from build123d import *

# Parameters (mm, degrees)
SKETCH2_W           = 250
SKETCH2_H           = 250
BOSS_EXTRUDE1_DEPTH = 3.175
SKETCH10_W          = 45
SKETCH10_H          = 3.175
BOSS_EXTRUDE2_DEPTH = 12.5
SKETCH11_W          = 45
SKETCH11_H          = 3.175
BOSS_EXTRUDE3_DEPTH = 12.5
SKETCH13_W          = 45
SKETCH13_H          = 3.175
BOSS_EXTRUDE4_DEPTH = 12.5
SKETCH14_W          = 45
SKETCH14_H          = 3.175
BOSS_EXTRUDE5_DEPTH = 12.5
M3_TAPPED_HOLE1_D   = 2.5
SKETCH21_R          = 1.25
CUT_EXTRUDE2_DEPTH  = 10
SKETCH23_R          = 2.9718
CUT_EXTRUDE10_DEPTH = 10


with BuildPart() as part:
    # Sketch2 → Boss-Extrude1 (new body)
    with BuildSketch(Plane(origin=(0, 0, 0), x_dir=(1, 0, 0), z_dir=(0, 1, 0))):
        Rectangle(SKETCH2_W, SKETCH2_H)
    extrude(amount=BOSS_EXTRUDE1_DEPTH)

    # Sketch10 → Boss-Extrude2 (add)
    with BuildSketch(Plane(origin=(0, 0, -125), x_dir=(-1, 0, 0), z_dir=(0, 0, -1))):
        with Locations((0, 1.5875)):
            Rectangle(SKETCH10_W, SKETCH10_H)
    extrude(amount=BOSS_EXTRUDE2_DEPTH)

    # Sketch11 → Boss-Extrude3 (add)
    with BuildSketch(Plane.ZY.offset(125)):
        with Locations((0, 1.5875)):
            Rectangle(SKETCH11_W, SKETCH11_H)
    extrude(amount=BOSS_EXTRUDE3_DEPTH)

    # Sketch13 → Boss-Extrude4 (add)
    with BuildSketch(Plane.XY.offset(125)):
        with Locations((0, 1.5875)):
            Rectangle(SKETCH13_W, SKETCH13_H)
    extrude(amount=BOSS_EXTRUDE4_DEPTH)

    # Sketch14 → Boss-Extrude5 (add)
    with BuildSketch(Plane(origin=(125, 0, 0), x_dir=(0, 0, -1), z_dir=(1, 0, 0))):
        with Locations((0, 1.5875)):
            Rectangle(SKETCH14_W, SKETCH14_H)
    extrude(amount=BOSS_EXTRUDE5_DEPTH)

    # M3 Tapped Hole1 (through all)
    with Locations(Plane(origin=(-115, 3.175, -115), x_dir=(0, 0, 1), z_dir=(0, 1, 0))):
        with Locations((0, 0)):
            Hole(M3_TAPPED_HOLE1_D / 2)

    # Sketch21 → Cut-Extrude2 (cut)
    with BuildSketch(Plane(origin=(0, 3.175, 0), x_dir=(1, 0, 0), z_dir=(0, 1, 0))):
        with Locations((115, 115)):
            Circle(SKETCH21_R)
        with Locations((115, -115)):
            Circle(SKETCH21_R)
        with Locations((-115, -115)):
            Circle(SKETCH21_R)
    extrude(amount=-CUT_EXTRUDE2_DEPTH, mode=Mode.SUBTRACT)

    # Sketch23 → Cut-Extrude10 (cut)
    with BuildSketch(Plane(origin=(0, 3.175, 0), x_dir=(1, 0, 0), z_dir=(0, 1, 0))):
        with Locations((-70.403440877, -69.85)):
            Circle(SKETCH23_R)
        with Locations((-70.403440877, 69.85)):
            Circle(SKETCH23_R)
        with Locations((69.296559123, 69.85)):
            Circle(SKETCH23_R)
        with Locations((69.296559123, -69.85)):
            Circle(SKETCH23_R)
    extrude(amount=-CUT_EXTRUDE10_DEPTH, mode=Mode.SUBTRACT)


solid = part.part
The model under review builds one solid part; all positions refer to its coordinate system, in mm. Round coordinates to 2 decimals unless told otherwise and drop trailing zeros. Loops run counter-clockwise (first coordinate to the right, second up) from the corner with the lowest first, then second, coordinate; pieces in that order, holes last. Notation, with made-up numbers: (36.25, -34.75) -> (41.25, -34.75) arc R20 ccw to (41.25, -12.75) -> close; hole circle Ø1 at (-15.75, -22). An arc over 180 degrees is marked (long way). Return JSON: item names as keys, results as strings.
(1) The part is to be moulded in two halves that separate along Z. For faces 1 (the cylindrical face through (-67.66, 1.61, 70.99)), 2 (the flat face through (-2, 3.175, -2)), say which applies: released by +Z, released by -Z, zero draft, split by the parting line, or undercut.
Solved:
{"face 1": "undercut", "face 2": "zero draft"}
(2) For line 1 (X direction, y = 1.3, z = 115); line 2 (X direction, y = 1.7, z = -69.85); line 3 (Z direction, x = -115.5, y = 1.35), list the stretches that pass through material, from the lowest coordinate up.
Solved:
{"line 1": "-125 to -116.25, -113.75 to 113.75, 116.25 to 125", "line 2": "-125 to -73.38, -67.43 to 66.32, 72.27 to 125", "line 3": "-125 to -116.15, -113.85 to 113.85, 116.15 to 125"}
(3) Add section A-A on y = 2.35. State how many separate pieces and enclosed holes the cut face has, plus the area to 3 significant figures.
Solved:
{"separate pieces": "1", "enclosed holes": "8", "area": "64,600 mm2"}
(4) Add section C-C on z = 48.5. Write out the cut boundary in (x, y) (3 decimals).
Solved:
{"outline": "(-125, 0) -> (125, 0) -> (125, 3.175) -> (-125, 3.175) -> close"}
(5) For pin 1 (1.6 mm diameter, centred on y = 1.5, z = -133, fed in from +X); pin 2 (1.5 mm diameter, centred on y = 3, z = -85.5, fed in from -X); pin 3 (5 mm diameter, centred on x = -70.4, z = -69.85, fed in from -Y); pin 4 (1.6 mm diameter, centred on y = 1.5, z = -96.5, fed in from +X), all flat-tipped, find the tip position at first contact; note any pin that passes through.
Solved:
{"pin 1": "x = 22.5", "pin 2": "x = -125", "pin 3": "through", "pin 4": "x = 125"}
(6) Add section B-B on x = -48. Write out the cut boundary in (y, z) (3 decimals).
Solved:
{"outline": "(0, -125) -> (3.175, -125) -> (3.175, 125) -> (0, 125) -> close"}
